from build123d import *

# Parameters (mm, degrees)
F3_DEPTH = 180
F5_DEPTH = 35
F6_SIZE  = 1


with BuildPart() as f1:
    # F0 (on Front) → F1 (revolve)
    with BuildSketch(Plane.XZ):
        Polygon((-302, 6.5), (-302, 0), (-185, 0), (175, 0), (218, 0), (218, 11.5), (214, 11.5), (214, 10.9), (212.7, 10.9), (212.7, 11.5), (185, 11.5), (185, 15), (-185, 15), (-185, 12.5), (-214, 12.5), (-214, 11.9), (-215.3, 11.9), (-215.3, 12.5), (-302, 12.5), align=None)
    revolve(axis=Axis((-5, 0, 0), (1, 0, 0)))

    # F2 (on Right) → F3 (cut, symmetric)
    with BuildSketch(Plane.YZ):
        with BuildLine():
            Line((-12.9903810568, -7.5), (-12.9903810568, 7.5))
            ThreePointArc((-12.9903810568, 7.5), (-15, 0), (-12.9903810568, -7.5))
        make_face()
        with BuildLine():
            ThreePointArc((12.9903810568, -7.5), (15, 0), (12.9903810568, 7.5))
            Line((12.9903810568, 7.5), (12.9903810568, -7.5))
        make_face()
    extrude(amount=F3_DEPTH, both=True, mode=Mode.SUBTRACT)

    # F4 (on face) → F5 (cut)
    with BuildSketch(Plane(origin=(-302, 0, 0), x_dir=(0, -1, 0), z_dir=(-1, 0, 0))):
        with BuildLine():
            Line((-10.5, -6.7823299831), (-10.5, 6.7823299831))
            ThreePointArc((-10.5, 6.7823299831), (-12.5, 0), (-10.5, -6.7823299831))
        make_face()
        with BuildLine():
            ThreePointArc((12.5, 0), (11.9895788083, 3.5355339059), (10.5, 6.7823299831))
            Line((10.5, 6.7823299831), (10.5, -6.7823299831))
            ThreePointArc((10.5, -6.7823299831), (11.9895788083, -3.5355339059), (12.5, 0))
        make_face()
    extrude(amount=-F5_DEPTH, mode=Mode.SUBTRACT)

    # F6
    f6_edges = [f1.edges().sort_by_distance(p)[0] for p in [
        (-185, 0, -15),
        (185, 0, -15),
        (218, 0, -11.5),
    ]]
    chamfer(f6_edges, length=F6_SIZE)


solid = f1.part
Input: part model. Units: mm. Frame: model coordinates. A direction names the side the tool comes from. Round coordinates to 2 decimals unless told otherwise and drop trailing zeros. Order: outer loops, then holes, each group sorted by start corner. A loop starts at its lowest first (then second) coordinate and runs counter-clockwise, first axis right, second up.
1. Cut plane B-B, the plane x = -193. Output: boundary loops of the cut face in (y, z).
The answers:
outline: circle Ø25 at (0, 0)
2. Set-up query: faces 4 (the face through (-249.624, -0.55, -12.488)), 5 (the face through (3, 12.99, 0)), 6 (the face through (-3, -12.99, 0)), 7 (the face through (-214, 5, 11)), 8 (the face through (215.5, -11.4, -1.5)). Return all of +Z, -Z, +X, -X, +Y, -Y with unobstructed straight access to the full face (end or side cutting, diameter ignored); none if empty.
The answers:
face 4: -X
face 5: +Z, -Z, +Y
face 6: +Z, -Z, -Y
face 7: none
face 8: +X
3. Material intervals for line 1 (X direction, y = 11, z = 4.75); line 2 (Y direction, x = -76, z = 6.5); line 3 (Y direction, x = -230, z = 10), sorted ascending.
The answers:
line 1: x = -267 to -215.3, -214 to 185
line 2: y = -12.99 to 12.99
line 3: y = -7.5 to 7.5
4. Cut plane C-C, the plane x = -51.5. Output: boundary loops of the cut face in (y, z), then the cut area to 3 significant figures.
The answers:
outline: (-12.99, -7.5) arc R15 ccw to (12.99, -7.5) - (12.99, 7.5) arc R15 ccw to (-12.99, 7.5) - close
area: 666 mm2
5. Mould query, pull axis X, two halves, no side actions, for faces 1 (the face through (-185, -11.5, -5.3)), 2 (the face through (-199.703, -3.755, 11.923)), 3 (the face through (213.34, -3.27, 10.4)). Classes: released by +X, released by -X, zero draft, split by the parting line, or undercut.
The answers:
face 1: released by -X
face 2: zero draft
face 3: undercut
6. Pin query (flat end, axial travel): P1, Ø2, axis at x = -147.5, z = -2.5, coming from the +Y side; P2, Ø1, axis at x = 36, y = 5, coming from the -Z side; P3, Ø15, axis at x = -292, z = 3, coming from the -Y side. Return the tip coordinate at first contact, or that it passes through.
The answers:
P1: stops at y = 12.99
P2: stops at z = -14.31
P3: stops at y = -10.5
